```python
from build123d import *

# Parameters (mm, degrees)
SKETCH1_W           = 50
SKETCH1_H           = 25
BOSS_EXTRUDE1_DEPTH = 20
SKETCH4_R           = 5
BOSS_EXTRUDE2_DEPTH = 50
CUT_EXTRUDE1_DEPTH  = 50


with BuildPart() as part:
    # Sketch1 → Boss-Extrude1 (new, symmetric)
    with BuildSketch(Plane.XY):
        with Locations((0, 12.5)):
            Rectangle(SKETCH1_W, SKETCH1_H)
    extrude(amount=BOSS_EXTRUDE1_DEPTH, both=True)

    # Sketch4 → Boss-Extrude2 (add)
    with BuildSketch(Plane(origin=(0, 25, 0), x_dir=(1, 0, 0), z_dir=(0, 1, 0))):
        with Locations(Location((0, 0, 0), (0, 0, 180))):
            Circle(SKETCH4_R)
    extrude(amount=BOSS_EXTRUDE2_DEPTH)

    # Sketch6 → Cut-Extrude1 (cut)
    with BuildSketch(Plane(origin=(25, 0, 0), x_dir=(0, 0, -1), z_dir=(1, 0, 0))):
        with BuildLine():
            ThreePointArc((5, 12.5), (3.535533906, 16.035533906), (0, 17.5))
            Line((0, 17.5), (0, 7.5))
            ThreePointArc((0, 7.5), (3.535533906, 8.964466094), (5, 12.5))
        make_face()
        with BuildLine():
            Line((0, 7.5), (0, 17.5))
            ThreePointArc((0, 17.5), (-5, 12.5), (0, 7.5))
        make_face()
    extrude(amount=-CUT_EXTRUDE1_DEPTH, mode=Mode.SUBTRACT)


solid = part.part
```
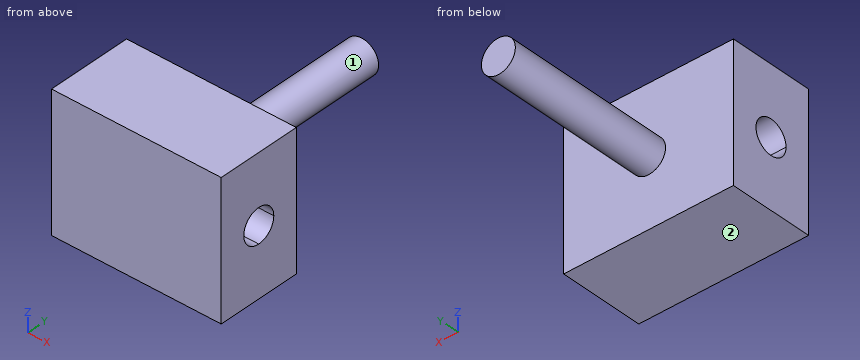
Build history of the part. All positions in model axes, mm. Face numbers are marked on the shaded views. A direction names the side the tool comes from. Coordinates: 2 decimals unless noted, no trailing zeros. Order: outer loops, then holes, each group sorted by start corner. A loop starts at its lowest first (then second) coordinate and runs counter-clockwise, first axis right, second up.
Item 1: Drill centre lines: L1, parallel to Y at x = 2, z = 14; L2, parallel to Y at x = -17, z = 4; L3, parallel to Y at x = 19, z = 3. Where is each one in solid material? Low to high.
Filled in:
L1: y = 0 to 25
L2: y = 0 to 9.5, 15.5 to 25
L3: y = 0 to 8.5, 16.5 to 25
Item 2: Saw through at B-B on z = 6. List the corners of the cut face in (x, y), then the cut area to 3 significant figures.
Filled in:
outline: (-25, 0) - (25, 0) - (25, 25) - (-25, 25) - close
area: 1,250 mm2
Item 3: Saw through at A-A on x = -19. List the corners of the cut face in (y, z), then the cut area to 3 significant figures.
Filled in:
outline: (0, -20) - (25, -20) - (25, 20) - (0, 20) - close; hole circle Ø10 at (12.5, 0)
area: 921 mm2
Item 4: Saw through at C-C on x = 0. List the corners of the cut face in (y, z).
Filled in:
outline: (0, -20) - (25, -20) - (25, -5) - (75, -5) - (75, 5) - (25, 5) - (25, 20) - (0, 20) - close; hole circle Ø10 at (12.5, 0)
Item 5: Tool access for the marked faces 1 and 2: list every direction of +Z, -Z, +X, -X, +Y, -Y with a clear straight run to the whole face (end or side of a thin tool).
Filled in:
face 1: +Y
face 2: -Z, +X, -X, +Y, -Y
Item 6: Saw through at D-D on y = 48. List the corners of the cut face in (x, z), then the cut area to 3 significant figures.
Filled in:
outline: circle Ø10 at (0, 0)
area: 78.5 mm2
Item 7: Drop flat-ended pins along their axis: pin 1 Ø1.5 at (x, y) = (5, 53) entering from -Z; pin 2 Ø10 at (y, z) = (31, 4) entering from -X; pin 3 Ø1 at (x, z) = (7, 7) entering from +Y. Give the stop position or say it passes through.
Filled in:
pin 1: stops at z = -2.63
pin 2: stops at x = -5
pin 3: stops at y = 25
